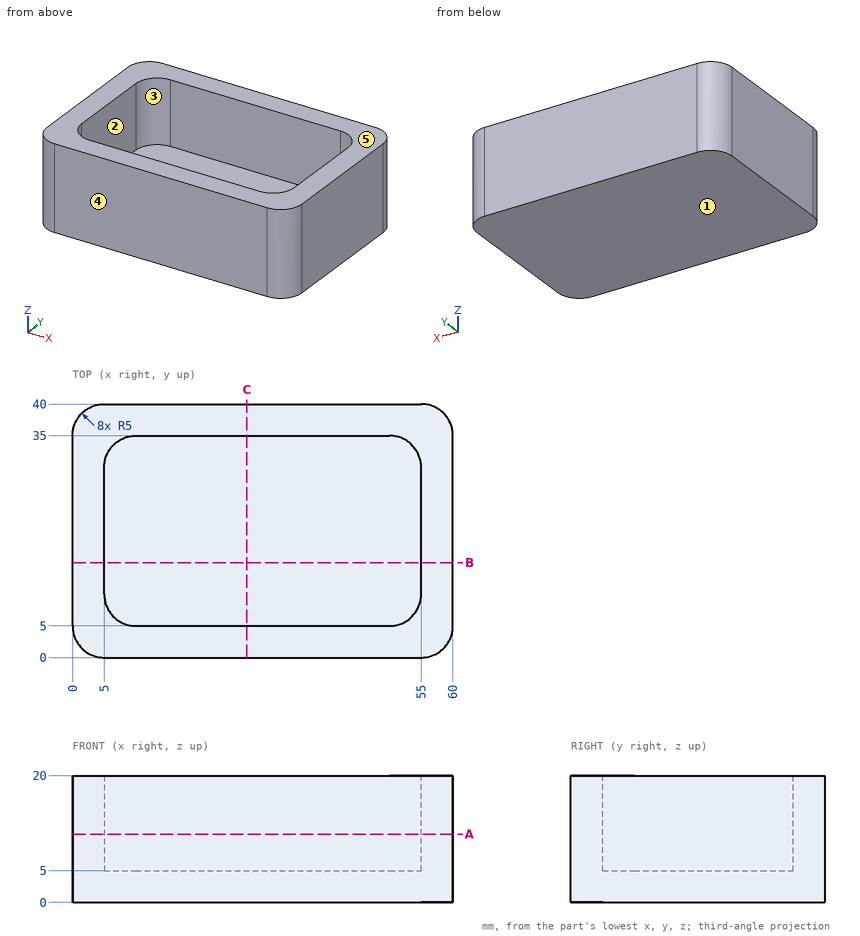
Geometry check sheet. Reference: drawing and pictorial views, mm from the part's lowest x, y, z. A direction names the side the tool comes from. Round coordinates to 2 decimals unless told otherwise and drop trailing zeros. Order: outer loops, then holes, each group sorted by start corner. A loop starts at its lowest first (then second) coordinate and runs counter-clockwise, first axis right, second up. Notation, with made-up numbers: M 13.25,-6 L 37.25,-6 A35 cw 37.25,31 Z; hole C 29,65 d10. An arc over 180 degrees is marked long. One line per item, written item: value. Start each with the question number.
1. Scan lines: line 1 along X through (y, z) = (13.5, 7.25); line 2 along Y through (x, z) = (10, 10.5); line 3 along Z through (x, y) = (13.5, 23). Record each from-to range of solid material in increasing order.
2. Release check for a two-part mould opening along Y. For the marked faces 3, 4 and 5 record: released by +Y, released by -Y, zero draft, split by the parting line, or undercut.
3. Section check C-C on x = 27.5. Enter the section's corners in (y, z).
4. Gauge pin test, flat ends, axial feed: P1, Ø3, axis at y = 25, z = 18, coming from the -X side; P2, Ø5, axis at x = 35.5, y = 32, coming from the +Z side. Record the tip position at first contact, or that the pin passes through.
5. Section check A-A on z = 10.75. Enter the section's corners in (x, y), and give its area (3 significant figures).
6. Section check B-B on y = 15. Enter the section's corners in (x, z).
7. Access from +Z, -Z, +X, -X, +Y, -Y to the whole of each face (thin tool, end or side, straight path). Record for the marked faces 1 and 2.
Results found:
1. line 1: 0 to 5, 55 to 60
1. line 2: 0 to 5, 35 to 40
1. line 3: 0 to 5
2. face 3: undercut
2. face 4: released by -Y
2. face 5: zero draft
3. outline: M 0,0 L 40,0 L 40,20 L 35,20 L 35,5 L 5,5 L 5,20 L 0,20 Z
4. P1: x = 0
4. P2: z = 5
5. outline: M 0,5 A5 ccw 5,0 L 55,0 A5 ccw 60,5 L 60,35 A5 ccw 55,40 L 5,40 A5 ccw 0,35 Z; hole M 5,10 A5 ccw 10,5 L 50,5 A5 ccw 55,10 L 55,30 A5 ccw 50,35 L 10,35 A5 ccw 5,30 Z
5. area: 900 mm^2
6. outline: M 0,0 L 60,0 L 60,20 L 55,20 L 55,5 L 5,5 L 5,20 L 0,20 Z
7. face 1: -Z, +X, -X, +Y, -Y
7. face 2: +Z
